Check sheet for the modelled part. Datum: model origin and axes. Units: mm. Face numbers are marked on the shaded views. A direction names the side the tool comes from. Give positions to 0.01 mm unless a question says otherwise; leave off trailing zeros. Write each loop counter-clockwise with the first axis right and the second up, starting at its lowest first coordinate (ties: lowest second). Pieces come first, ordered by that corner, then holes. Notation, with made-up numbers: M 29,60 L 60,60 A5 cw 60,65 Z; hole C 16.25,79 d6. An arc over 180 degrees is marked long. Write item = value, one per line. Start each with the question number.
1) Cross-section at A-A, the plane x = 43.5. Record the cut outline in (y, z).
2) Cross-section at D-D, the plane x = -1. Record the cut outline in (y, z).
3) Cross-section at C-C, the plane z = 5.5. Record the cut outline in (x, y).
4) Cross-section at B-B, the plane y = 1. Record the cut outline in (x, z), plus the area to 3 significant figures.
5) Access from +Z, -Z, +X, -X, +Y, -Y to the whole of each face (thin tool, end or side, straight path). Record for the marked faces 1 and 2.
6) Mould release check, pull along Y, two halves, no side actions. Record for the marked faces 3, 4, 5 and 6: released by +Y, released by -Y, zero draft, split by the parting line, or undercut.
7) Scan lines: line 1 along Z through (x, y) = (29.5, -1); line 2 along Y through (x, z) = (-28.5, -16.5). Record each from-to range of solid material in increasing order. Write a range as [from, to].
```python
from build123d import *

# Parameters (mm, degrees)
SKETCH1_W           = 38.1
SKETCH1_H           = 38.1
SKETCH1_W_2         = 33.8836
SKETCH1_H_2         = 33.8836
BOSS_EXTRUDE1_DEPTH = 50.8
FILLET1_R           = 2.54
SKETCH3_R           = 16.764
CUT_EXTRUDE2_DEPTH  = 67.295946332
CUT_EXTRUDE3_DEPTH  = 67.295946494


with BuildPart() as part:
    # Sketch1 → Boss-Extrude1 (new, symmetric)
    with BuildSketch(Plane(origin=(0, 0, 0), x_dir=(0, 0, -1), z_dir=(1, 0, 0))):
        Rectangle(SKETCH1_W, SKETCH1_H)
        Rectangle(SKETCH1_W_2, SKETCH1_H_2, mode=Mode.SUBTRACT)
    extrude(amount=BOSS_EXTRUDE1_DEPTH, both=True)

    # Fillet1
    fillet1_edges = [part.edges().sort_by_distance(p)[0] for p in [
        (0, -16.9418, -16.9418),
        (0, 16.9418, -16.9418),
        (0, 16.9418, 16.9418),
        (0, -16.9418, 16.9418),
        (0, 19.05, 19.05),
        (0, 19.05, -19.05),
        (0, -19.05, -19.05),
        (0, -19.05, 19.05),
    ]]
    fillet(fillet1_edges, radius=FILLET1_R)

    # Sketch3 → Cut-Extrude2 (cut, through all)
    with BuildSketch(Plane(origin=(0, 19.05, 0), x_dir=(1, 0, 0), z_dir=(0, 1, 0))):
        with Locations(Location((0, 0, 0), (0, 0, 279.986551447))):
            Circle(SKETCH3_R)
    extrude(amount=-CUT_EXTRUDE2_DEPTH, mode=Mode.SUBTRACT)

    # Sketch4 → Cut-Extrude3 (cut, through all)
    with BuildSketch(Plane(origin=(0, 19.05, 0), x_dir=(1, 0, 0), z_dir=(0, 1, 0))):
        with BuildLine():
            Line((-45.72, 19.05), (-50.8, 19.05))
            Line((-50.8, 19.05), (-50.8, -19.05))
            Line((-50.8, -19.05), (-45.72, -19.05))
            ThreePointArc((-45.72, -19.05), (-49.53, 0), (-45.72, 19.05))
        make_face()
        with BuildLine():
            Line((50.8, 16.51), (46.69733183, 16.51))
            ThreePointArc((46.69733183, 16.51), (48.81669666, 8.375621006), (49.53, 0))
            ThreePointArc((49.53, 0), (48.81669666, -8.375621006), (46.69733183, -16.51))
            Line((46.69733183, -16.51), (50.8, -16.51))
            Line((50.8, -16.51), (50.8, 16.51))
        make_face()
        with BuildLine():
            Line((50.8, 19.05), (45.72, 19.05))
            ThreePointArc((45.72, 19.05), (46.226114974, 17.786713985), (46.69733183, 16.51))
            Line((46.69733183, 16.51), (50.8, 16.51))
            Line((50.8, 16.51), (50.8, 19.05))
        make_face()
        with BuildLine():
            ThreePointArc((46.69733183, -16.51), (46.226114974, -17.786713985), (45.72, -19.05))
            Line((45.72, -19.05), (50.8, -19.05))
            Line((50.8, -19.05), (50.8, -16.51))
            Line((50.8, -16.51), (46.69733183, -16.51))
        make_face()
    extrude(amount=-CUT_EXTRUDE3_DEPTH, mode=Mode.SUBTRACT)


solid = part.part
```
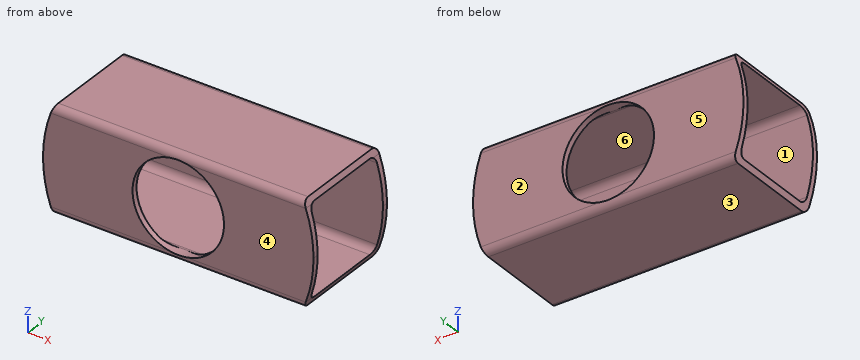
Reply:
q1.outline = M -19.05,-16.51 A2.54 ccw -16.51,-19.05 L 16.51,-19.05 A2.54 ccw 19.05,-16.51 L 19.05,16.51 A2.54 ccw 16.51,19.05 L -16.51,19.05 A2.54 ccw -19.05,16.51 Z; hole M -16.94,-14.4 A2.54 ccw -14.4,-16.94 L 14.4,-16.94 A2.54 ccw 16.94,-14.4 L 16.94,14.4 A2.54 ccw 14.4,16.94 L -14.4,16.94 A2.54 ccw -16.94,14.4 Z
q2.outline = M -19.04,-16.73 A2.54 ccw -16.51,-19.05 L 16.51,-19.05 A2.54 ccw 19.04,-16.73 L 15.41,-16.73 A2.54 cw 14.4,-16.94 L -14.4,-16.94 A2.54 cw -15.41,-16.73 Z; M -19.04,16.73 L -15.41,16.73 A2.54 cw -14.4,16.94 L 14.4,16.94 A2.54 cw 15.41,16.73 L 19.04,16.73 A2.54 ccw 16.51,19.05 L -16.51,19.05 A2.54 ccw Z
q3.outline = M -49.22,-19.05 L -15.84,-19.05 L -15.84,-16.94 L -49.22,-16.94 Z; M -49.22,16.94 L -15.84,16.94 L -15.84,19.05 L -49.22,19.05 Z; M 15.84,-19.05 L 49.22,-19.05 L 49.22,-16.94 L 15.84,-16.94 Z; M 15.84,16.94 L 49.22,16.94 L 49.22,19.05 L 15.84,19.05 Z
q4.outline = M -46.54,-16.94 A49.53 ccw -45.72,-19.05 L 45.72,-19.05 A49.53 ccw 46.54,-16.94 Z; M -46.54,16.94 L 46.54,16.94 A49.53 ccw 45.72,19.05 L -45.72,19.05 A49.53 ccw Z
q4.area = 389 mm2
q5.face_1 = +X, -X
q5.face_2 = +Z, -Z, +X, -X, +Y
q6.face_3 = zero draft
q6.face_4 = released by -Y
q6.face_5 = released by +Y
q6.face_6 = undercut
q7.line_1 = [-19.05, -16.94], [16.94, 19.05]
q7.line_2 = [-19.05, -15.83], [15.83, 19.05]
